```python
from build123d import *

# Parameters (mm, degrees)
BOSS_EXTRUDE1_DEPTH           = 2.54
BOSS_EXTRUDE2_DEPTH           = 2.54
BOSS_EXTRUDE2_DEPTH_BACK      = 5.08
HOLE1_OUTLINE_R               = 11.43
HOLE1_DEPTH                   = 2.54
CSK_FOR_M3_SFHCS1_D           = 3.6
CSK_FOR_M3_SFHCS1_CSINK_D     = 6.72
CSK_FOR_M3_SFHCS1_CSINK_ANGLE = 90
SKETCH9_W                     = 1.8288
SKETCH9_H                     = 5.08
F_6_CLEARANCE_HOLE_AT_2_COUNT = 2
F_6_CLEARANCE_HOLE_AT_2_PITCH = 55.444204897
F_6_CLEARANCE_HOLE_AT_3_COUNT = 2
F_6_CLEARANCE_HOLE_AT_3_PITCH = 104.402947299
F_6_CLEARANCE_HOLE_AT_4_COUNT = 2
F_6_CLEARANCE_HOLE_AT_4_PITCH = 88.464204897
BOSS_EXTRUDE4_START           = -5.08
SKETCH10_R                    = 1.8288
BOSS_EXTRUDE4_DEPTH           = 7.62
FILLET4_R                     = 2.54
SKETCH11_R                    = 3.175
BOSS_EXTRUDE5_DEPTH           = 3.175
TAP_DRILL_FOR_4_40_TAP1_D     = 2.2606
TAP_DRILL_FOR_4_40_TAP1_DEPTH = 5.08
TAP_DRILL_FOR_4_40_TAP1_TIP   = 0.679152758
SKETCH14_R                    = 1.8288
CUT_EXTRUDE1_DEPTH            = 62.843262568
CUT_EXTRUDE2_DEPTH            = 62.500004065


# Read off the part's stored shape, not the designer's step: Hole1
with BuildPart() as part:
    # Sketch1 → Boss-Extrude1 (new body)
    with BuildSketch(Plane(origin=(0, 0, 0), x_dir=(1, 0, 0), z_dir=(0, 1, 0))):
        with BuildLine():
            Line((40.64, -34.29), (-40.64, -34.29))
            ThreePointArc((-40.64, -34.29), (-47.824204897, -31.314204897), (-50.8, -24.13))
            Line((-50.8, -24.13), (-50.8, 24.13))
            ThreePointArc((-50.8, 24.13), (-47.824204897, 31.314204897), (-40.64, 34.29))
            Line((-40.64, 34.29), (40.64, 34.29))
            ThreePointArc((40.64, 34.29), (47.824204897, 31.314204897), (50.8, 24.13))
            Line((50.8, 24.13), (50.8, -24.13))
            ThreePointArc((50.8, -24.13), (47.824204897, -31.314204897), (40.64, -34.29))
        make_face()
    extrude(amount=BOSS_EXTRUDE1_DEPTH)

    # Sketch2 → Boss-Extrude2 (add, two sides: drawn at the far end of the back side and taken through both)
    with BuildSketch(Plane.XZ.offset(-BOSS_EXTRUDE2_DEPTH_BACK)):
        with BuildLine():
            Line((48.133, -24.13), (48.133, 24.13))
            ThreePointArc((48.133, 24.13), (45.938351111, 29.428351111), (40.64, 31.623))
            Line((40.64, 31.623), (-40.64, 31.623))
            ThreePointArc((-40.64, 31.623), (-45.938351111, 29.428351111), (-48.133, 24.13))
            Line((-48.133, 24.13), (-48.133, -24.13))
            ThreePointArc((-48.133, -24.13), (-45.938351111, -29.428351111), (-40.64, -31.623))
            Line((-40.64, -31.623), (40.64, -31.623))
            ThreePointArc((40.64, -31.623), (45.938351111, -29.428351111), (48.133, -24.13))
        make_face()
        with BuildLine():
            Line((45.593, -24.13), (45.593, 24.13))
            ThreePointArc((45.593, 24.13), (44.142299887, 27.632299887), (40.64, 29.083))
            Line((40.64, 29.083), (-40.64, 29.083))
            ThreePointArc((-40.64, 29.083), (-44.142299887, 27.632299887), (-45.593, 24.13))
            Line((-45.593, 24.13), (-45.593, -24.13))
            ThreePointArc((-45.593, -24.13), (-44.142299887, -27.632299887), (-40.64, -29.083))
            Line((-40.64, -29.083), (40.64, -29.083))
            ThreePointArc((40.64, -29.083), (44.142299887, -27.632299887), (45.593, -24.13))
        make_face(mode=Mode.SUBTRACT)
    extrude(amount=BOSS_EXTRUDE2_DEPTH + BOSS_EXTRUDE2_DEPTH_BACK)

    # Hole1 outline → Hole1 (cut)
    with BuildSketch(Plane(origin=(0, 0, 0), x_dir=(1, 0, 0), z_dir=(0, 1, 0))):
        with Locations((-25.146, 0)):
            Circle(HOLE1_OUTLINE_R)
    extrude(amount=HOLE1_DEPTH, mode=Mode.SUBTRACT)

    # CSK for M3 SFHCS1 (through all)
    with Locations(Plane(origin=(48.934573601, 0, -16.825198342), x_dir=(0, 0, 1), z_dir=(0, -1, 0))):
        with Locations((32.325198342, 89.580573601), (1.325198342, 89.580573601), (1.325198342, 57.850841183), (32.325198342, 58.580573601)):
            CounterSinkHole(CSK_FOR_M3_SFHCS1_D / 2, CSK_FOR_M3_SFHCS1_CSINK_D / 2, counter_sink_angle=CSK_FOR_M3_SFHCS1_CSINK_ANGLE)

    # Sketch9 → #6 Clearance Hole (revolve, cut)
    with BuildSketch(Plane(origin=(44.232102448, 2.54, -27.722102448), x_dir=(0, 0, 1), z_dir=(1, 0, 0))):
        with Locations((0.9144, 2.54)):
            Rectangle(SKETCH9_W, SKETCH9_H)
    f_6_clearance_hole = revolve(axis=Axis((44.232102448, 8.89, -27.722102448), (0, -1, 0)), mode=Mode.SUBTRACT)

    # #6 Clearance Hole at 2: #6 Clearance Hole ×2
    with Locations(*[(0, 0, i * F_6_CLEARANCE_HOLE_AT_2_PITCH) for i in range(1, F_6_CLEARANCE_HOLE_AT_2_COUNT)]):
        add(f_6_clearance_hole, mode=Mode.SUBTRACT)

    # #6 Clearance Hole at 3: #6 Clearance Hole ×2
    with Locations(*[Vector(-0.8473343634990179, 0, 0.5310597672896286) * (i * F_6_CLEARANCE_HOLE_AT_3_PITCH) for i in range(1, F_6_CLEARANCE_HOLE_AT_3_COUNT)]):
        add(f_6_clearance_hole, mode=Mode.SUBTRACT)

    # #6 Clearance Hole at 4: #6 Clearance Hole ×2
    with Locations(*[(-i * F_6_CLEARANCE_HOLE_AT_4_PITCH, 0, 0) for i in range(1, F_6_CLEARANCE_HOLE_AT_4_COUNT)]):
        add(f_6_clearance_hole, mode=Mode.SUBTRACT)

    # Sketch10 → Boss-Extrude4 (add)
    # profile 1 of 4: a face of its own
    with BuildSketch(Plane.XZ.offset(BOSS_EXTRUDE4_START)):
        with BuildLine():
            ThreePointArc((-42.196740764, 31.45950252), (-45.938351111, 29.428351111), (-47.96950252, 25.686740764))
            ThreePointArc((-47.96950252, 25.686740764), (-41.222878588, 24.712878588), (-42.196740764, 31.45950252))
        make_face()
        with Locations(Location((-44.232102448, 27.722102448, 0), (0, 0, 90))):
            Circle(SKETCH10_R, mode=Mode.SUBTRACT)
    # profile 2 of 4: a face of its own
    with BuildSketch(Plane.XZ.offset(BOSS_EXTRUDE4_START)):
        with BuildLine():
            ThreePointArc((47.96950252, 25.686740764), (41.222878588, 24.712878588), (42.196740764, 31.45950252))
            ThreePointArc((42.196740764, 31.45950252), (45.938351111, 29.428351111), (47.96950252, 25.686740764))
        make_face()
        with Locations(Location((44.232102448, 27.722102448, 0), (0, 0, 90))):
            Circle(SKETCH10_R, mode=Mode.SUBTRACT)
    # profile 3 of 4: a face of its own
    with BuildSketch(Plane.XZ.offset(BOSS_EXTRUDE4_START)):
        with BuildLine():
            ThreePointArc((42.196740764, -31.45950252), (45.938351111, -29.428351111), (47.96950252, -25.686740764))
            ThreePointArc((47.96950252, -25.686740764), (41.222878588, -24.712878588), (42.196740764, -31.45950252))
        make_face()
        with Locations(Location((44.232102448, -27.722102448, 0), (0, 0, 90))):
            Circle(SKETCH10_R, mode=Mode.SUBTRACT)
    # profile 4 of 4: a face of its own
    with BuildSketch(Plane.XZ.offset(BOSS_EXTRUDE4_START)):
        with BuildLine():
            ThreePointArc((-47.96950252, -25.686740764), (-41.222878588, -24.712878588), (-42.196740764, -31.45950252))
            ThreePointArc((-42.196740764, -31.45950252), (-45.938351111, -29.428351111), (-47.96950252, -25.686740764))
        make_face()
        with Locations(Location((-44.232102448, -27.722102448, 0), (0, 0, 90))):
            Circle(SKETCH10_R, mode=Mode.SUBTRACT)
    extrude(amount=BOSS_EXTRUDE4_DEPTH)

    # Fillet4
    fillet4_edges = [part.edges().sort_by_distance(p)[0] for p in [
        (-40.199880439, 3.81, 29.083),
        (-45.593, 3.81, 23.689880439),
        (-45.593, -1.27, 23.689880439),
        (-40.199880439, -1.27, 29.083),
        (40.199880439, -1.27, 29.083),
        (45.593, -1.27, 23.689880439),
        (40.199880439, 3.81, 29.083),
        (45.593, 3.81, 23.689880439),
        (45.593, -1.27, -23.689880439),
        (40.199880439, -1.27, -29.083),
        (45.593, 3.81, -23.689880439),
        (40.199880439, 3.81, -29.083),
        (-40.199880439, -1.27, -29.083),
        (-45.593, -1.27, -23.689880439),
        (-40.199880439, 3.81, -29.083),
        (-45.593, 3.81, -23.689880439),
    ]]
    fillet(fillet4_edges, radius=FILLET4_R)

    # Sketch11 → Boss-Extrude5 (add)
    with BuildSketch(Plane(origin=(0, 2.54, 0), x_dir=(1, 0, 0), z_dir=(0, 1, 0))):
        with Locations(Location((38.1, 18.669, 0), (0, 0, 90))):
            Circle(SKETCH11_R)
        with Locations(Location((1.27, 18.669, 0), (0, 0, 90))):
            Circle(SKETCH11_R)
        with Locations(Location((1.27, -18.669, 0), (0, 0, 90))):
            Circle(SKETCH11_R)
        with Locations(Location((38.1, -18.669, 0), (0, 0, 90))):
            Circle(SKETCH11_R)
    extrude(amount=BOSS_EXTRUDE5_DEPTH)

    # Tap Drill for #4-40 Tap1
    with Locations(Plane(origin=(0, 5.715, 0), x_dir=(1, 0, 0), z_dir=(0, 1, 0))):
        with Locations((38.1, 18.669), (1.27, 18.669), (1.27, -18.669), (38.1, -18.669)):
            Hole(TAP_DRILL_FOR_4_40_TAP1_D / 2, depth=TAP_DRILL_FOR_4_40_TAP1_DEPTH)
            with Locations((0, 0, -(TAP_DRILL_FOR_4_40_TAP1_DEPTH + TAP_DRILL_FOR_4_40_TAP1_TIP / 2))):  # 118° drill point
                Cone(0, TAP_DRILL_FOR_4_40_TAP1_D / 2, TAP_DRILL_FOR_4_40_TAP1_TIP, mode=Mode.SUBTRACT)

    # Sketch14 → Cut-Extrude1 (cut, through all)
    with BuildSketch(Plane.XZ.offset(2.54)):
        with Locations(Location((44.232102448, -27.722102448, 0), (0, 0, 90))):
            Circle(SKETCH14_R)
        with Locations(Location((-44.232102448, -27.722102448, 0), (0, 0, 90))):
            Circle(SKETCH14_R)
        with Locations(Location((-44.232102448, 27.722102448, 0), (0, 0, 90))):
            Circle(SKETCH14_R)
        with Locations(Location((44.232102448, 27.722102448, 0), (0, 0, 90))):
            Circle(SKETCH14_R)
    extrude(amount=-CUT_EXTRUDE1_DEPTH, mode=Mode.SUBTRACT)

    # Sketch15 → Cut-Extrude2 (cut, through all)
    with BuildSketch(Plane(origin=(0, 2.54, 0), x_dir=(1, 0, 0), z_dir=(0, 1, 0))):
        with BuildLine():
            Line((-42.989587083, -21.5), (-7.302412917, -21.5))
            ThreePointArc((-7.302412917, -21.5), (-5.389436534, -19.756563466), (-3.646, -17.843587083))
            Line((-3.646, -17.843587083), (-3.646, 17.843587083))
            ThreePointArc((-3.646, 17.843587083), (-5.389436534, 19.756563466), (-7.302412917, 21.5))
            Line((-7.302412917, 21.5), (-42.989587083, 21.5))
            ThreePointArc((-42.989587083, 21.5), (-44.902563466, 19.756563466), (-46.646, 17.843587083))
            Line((-46.646, 17.843587083), (-46.646, -17.843587083))
            ThreePointArc((-46.646, -17.843587083), (-44.902563466, -19.756563466), (-42.989587083, -21.5))
        make_face()
    extrude(amount=CUT_EXTRUDE2_DEPTH, mode=Mode.SUBTRACT)


solid = part.part
```
Work out the finished part from the listing and answer in its coordinate system (mm). A direction names the side the tool comes from. Round coordinates to 2 decimals unless told otherwise and drop trailing zeros. Loops run counter-clockwise (first coordinate to the right, second up) from the corner with the lowest first, then second, coordinate; pieces in that order, holes last.
(1) For faces 4 (the flat face through (1, 4, 29.083)), 5 (the flat face through (-48.133, -1, 0)), 6 (the cylindrical face through (45.996, -1.252, 29.37)), 7 (the flat face through (38, 5.715, -20)), 8 (the flat face through (1, -1, 29.083)), determine the directions among +Z, -Z, +X, -X, +Y, -Y from which every point of the face is accessible in a straight line to the end or side of a thin tool.
Computed values:
face 4: +Y
face 5: +Z, -Z, -X, -Y
face 6: +Z, +X, -Y
face 7: +Z, -Z, +X, -X, +Y
face 8: -Y
(2) Each of these flat-tipped pins is pushed along its axis until it touches: P1, Ø2, axis at x = 38.1, z = -18.669, coming from the +Y side; P2, Ø6, axis at x = -44.23, z = -27.72, coming from the +Y side; P3, Ø8, axis at x = 15.5, z = 8, coming from the -Y side; P4, Ø2, axis at x = 44.23, z = -27.72, coming from the -Y side. Where does it stop, or does it pass through?
Computed values:
P1: stops at y = 0.56
P2: stops at y = 5.08
P3: stops at y = 0
P4: passes through
(3) Find the intervals of material crossed by L1, parallel to X at y = 0.95, z = 0; L2, parallel to X at y = -0.25, z = 3.5; L3, parallel to Z at x = -24, y = -1.25, in increasing order.
Computed values:
L1: x = -50.8 to -36.58, -13.72 to 50.8
L2: x = -48.13 to -45.59, 45.59 to 48.13
L3: z = -31.62 to -29.08, 29.08 to 31.62
(4) The part is cut by section B-B, the plane x = -28.5. Give the vertices of the cut face in (y, z).
Computed values:
outline: (-2.54, -31.62) - (0, -31.62) - (0, -34.29) - (2.54, -34.29) - (2.54, -31.62) - (5.08, -31.62) - (5.08, -29.08) - (2.54, -29.08) - (2.54, -10.93) - (0, -10.93) - (0, -29.08) - (-2.54, -29.08) - close; (-2.54, 29.08) - (0, 29.08) - (0, 10.93) - (2.54, 10.93) - (2.54, 29.08) - (5.08, 29.08) - (5.08, 31.62) - (2.54, 31.62) - (2.54, 34.29) - (0, 34.29) - (0, 31.62) - (-2.54, 31.62) - close
(5) The part is cut by section A-A, the plane z = 0. Give the vertices of the cut face in (x, y), and give its area (3 significant figures).
Computed values:
outline: (-50.8, 0) - (-48.13, 0) - (-48.13, -2.54) - (-45.59, -2.54) - (-45.59, 0) - (-36.58, 0) - (-36.58, 2.54) - (-46.65, 2.54) - (-46.65, 5.08) - (-48.13, 5.08) - (-48.13, 2.54) - (-50.8, 2.54) - close; (-13.72, 0) - (45.59, 0) - (45.59, -2.54) - (48.13, -2.54) - (48.13, 0) - (50.8, 0) - (50.8, 2.54) - (48.13, 2.54) - (48.13, 5.08) - (45.59, 5.08) - (45.59, 2.54) - (-13.72, 2.54) - close
area: 223 mm2
(6) The mould has two halves that part along X. Classify faces 1 (the cylindrical face through (45.88, -1.252, -29.486)), 2 (the cylindrical face through (-42.43, 2.06, 15.73)), 3 (the flat face through (0, -2.54, 31)): pulls with the +X half, pulls with the -X half, needs draft (parallel to the pull), parting line crosses it, or undercut.
Computed values:
face 1: pulls with the +X half
face 2: undercut
face 3: needs draft
